Check sheet for the modelled part. Datum: model origin and axes. Units: mm. Face numbers are marked on the shaded views. A direction names the side the tool comes from. Give positions to 0.01 mm unless a question says otherwise; leave off trailing zeros. Order: outer loops, then holes, each group sorted by start corner. A loop starts at its lowest first (then second) coordinate and runs counter-clockwise, first axis right, second up. Notation, with made-up numbers: (33.5, -39.5) - (42.5, -39.5) arc R16 cw to (42.5, -12.5) - close; hole circle Ø8 at (-1, 45.5). An arc over 180 degrees is marked (long way). Answer in a Markdown table with one row per item.
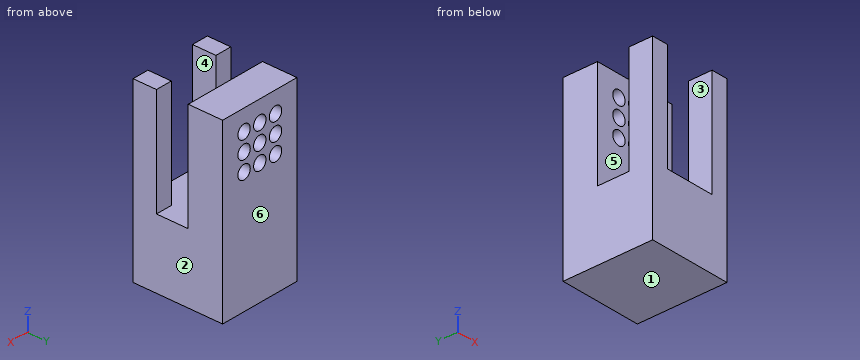
from build123d import *

# Parameters (mm, degrees)
SKETCH1_W           = 12
SKETCH1_H           = 10
SKETCH1_H_2         = 15.68
SKETCH1_R           = 1
BOSS_EXTRUDE1_DEPTH = 5
SKETCH1_3_W         = 12
SKETCH1_3_H         = 10
BOSS_EXTRUDE2_DEPTH = 8
SKETCH2_W           = 2.4
SKETCH2_H           = 3.4
BOSS_EXTRUDE3_DEPTH = 15.68


with BuildPart() as part:
    # Sketch1 → Boss-Extrude1 (new body)
    # profile 1 of 2: a face of its own
    with BuildSketch(Plane(origin=(0, 0, 0), x_dir=(1, 0, 0), z_dir=(0, 1, 0))):
        with Locations((0, 15.14)):
            Rectangle(SKETCH1_W, SKETCH1_H)
    # profile 2 of 2: a face of its own
    with BuildSketch(Plane(origin=(0, 0, 0), x_dir=(1, 0, 0), z_dir=(0, 1, 0))):
        with Locations((0, 2.3)):
            Rectangle(SKETCH1_W, SKETCH1_H_2)
        with Locations(Location((-2.54, -2.54, 0), (0, 0, 270))):
            Circle(SKETCH1_R, mode=Mode.SUBTRACT)
        with Locations(Location((-2.54, 0, 0), (0, 0, 270))):
            Circle(SKETCH1_R, mode=Mode.SUBTRACT)
        with Locations(Location((0, 0, 0), (0, 0, 270))):
            Circle(SKETCH1_R, mode=Mode.SUBTRACT)
        with Locations(Location((-2.54, 2.54, 0), (0, 0, 270))):
            Circle(SKETCH1_R, mode=Mode.SUBTRACT)
        with Locations(Location((0, 2.54, 0), (0, 0, 270))):
            Circle(SKETCH1_R, mode=Mode.SUBTRACT)
        with Locations(Location((0, -2.54, 0), (0, 0, 270))):
            Circle(SKETCH1_R, mode=Mode.SUBTRACT)
        with Locations(Location((2.54, -2.54, 0), (0, 0, 270))):
            Circle(SKETCH1_R, mode=Mode.SUBTRACT)
        with Locations(Location((2.54, 0, 0), (0, 0, 270))):
            Circle(SKETCH1_R, mode=Mode.SUBTRACT)
        with Locations(Location((2.54, 2.54, 0), (0, 0, 270))):
            Circle(SKETCH1_R, mode=Mode.SUBTRACT)
    extrude(amount=BOSS_EXTRUDE1_DEPTH)

    # Sketch1<3> → Boss-Extrude2 (add)
    with BuildSketch(Plane(origin=(0, 0, 0), x_dir=(1, 0, 0), z_dir=(0, 1, 0))):
        with Locations((0, 15.14)):
            Rectangle(SKETCH1_3_W, SKETCH1_3_H)
    extrude(amount=-BOSS_EXTRUDE2_DEPTH)

    # Sketch2 → Boss-Extrude3 (add)
    with BuildSketch(Plane.XY.offset(-10.14)):
        with Locations((-4.8, -6.3)):
            Rectangle(SKETCH2_W, SKETCH2_H)
        with Locations((4.8, -6.3)):
            Rectangle(SKETCH2_W, SKETCH2_H)
    extrude(amount=BOSS_EXTRUDE3_DEPTH)


solid = part.part
(1) Cross-section at D-D, the plane x = -4. Record the cut outline in (y, z), then the cut area to 3 significant figures.
Geometry says:
| item | result |
|---|---|
| outline | (-8, -20.14) - (5, -20.14) - (5, 5.54) - (0, 5.54) - (0, -10.14) - (-4.6, -10.14) - (-4.6, 5.54) - (-8, 5.54) - close |
| area | 262 mm² |
(2) Access from +Z, -Z, +X, -X, +Y, -Y to the whole of each face (thin tool, end or side, straight path). Record for the marked faces 4, 5 and 6.
Geometry says:
| item | result |
|---|---|
| face 4 | +Z, -Y |
| face 5 | +Z, +X, -X |
| face 6 | +Z, -Z, +X, -X, +Y |
(3) Cross-section at A-A, the plane z = -2.54. Record the cut outline in (x, y).
Geometry says:
| item | result |
|---|---|
| outline | (-6, -8) - (-3.6, -8) - (-3.6, -4.6) - (-6, -4.6) - close; (-6, 0) - (-3.54, 0) - (-3.54, 5) - (-6, 5) - close; (-1.54, 0) - (-1, 0) - (-1, 5) - (-1.54, 5) - close; (1, 0) - (1.54, 0) - (1.54, 5) - (1, 5) - close; (3.54, 0) - (6, 0) - (6, 5) - (3.54, 5) - close; (3.6, -8) - (6, -8) - (6, -4.6) - (3.6, -4.6) - close |
(4) Cross-section at C-C, the plane y = 4.25. Give the number of separate pieces and of enclosed holes in the cut face, then the cut area to 3 significant figures.
Geometry says:
| item | result |
|---|---|
| separate pieces | 1 |
| enclosed holes | 9 |
| area | 280 mm² |
(5) Cross-section at B-B, the plane x = 0. Record the cut outline in (y, z), then the cut area to 3 significant figures.
Geometry says:
| item | result |
|---|---|
| outline | (-8, -20.14) - (5, -20.14) - (5, -3.54) - (0, -3.54) - (0, -10.14) - (-8, -10.14) - close; (0, -1.54) - (5, -1.54) - (5, -1) - (0, -1) - close; (0, 1) - (5, 1) - (5, 1.54) - (0, 1.54) - close; (0, 3.54) - (5, 3.54) - (5, 5.54) - (0, 5.54) - close |
| area | 178 mm² |
(6) Thickness scan on L1, parallel to X at y = 3.5, z = -2.54; L2, parallel to Y at x = 4.25, z = 2.75; L3, parallel to X at y = -6.25, z = -5.5. Record the ranges inside material, lowest first.
Geometry says:
| item | result |
|---|---|
| L1 | -6 to -3.54, -1.54 to -1, 1 to 1.54, 3.54 to 6 |
| L2 | -8 to -4.6, 0 to 5 |
| L3 | -6 to -3.6, 3.6 to 6 |
(7) Gauge pin test, flat ends, axial feed: P1, Ø4, axis at y = -0.5, z = -2, coming from the +X side; P2, Ø4, axis at x = 1.5, y = -3, coming from the +Z side. Record the tip position at first contact, or that the pin passes through.
Geometry says:
| item | result |
|---|---|
| P1 | x = 6 |
| P2 | z = -10.14 |
(8) Mould release check, pull along X, two halves, no side actions. Record for the marked faces 1, 2 and 3: pulls with the +X half, pulls with the -X half, needs draft (parallel to the pull), parting line crosses it, or undercut.
Geometry says:
| item | result |
|---|---|
| face 1 | needs draft |
| face 2 | pulls with the +X half |
| face 3 | undercut |
